Source: three-view drawing plus pictorial views. Frame: mm from the lowest corner of the part. A direction names the side the tool comes from. Coordinates: 2 decimals unless noted, no trailing zeros. Order: outer loops, then holes, each group sorted by start corner. A loop starts at its lowest first (then second) coordinate and runs counter-clockwise, first axis right, second up. Notation, with made-up numbers: (72, 73.25) -> (130, 73.25) arc R17 cw to (130, 83.25) -> close; hole circle Ø2 at (43.5, 13). An arc over 180 degrees is marked (long way). Use one line per item in the form item = value. Start each with the question number.
1) Ray query, line 1 along Y through (x, z) = (6.25, 9.25) (1 decimal); line 2 along Y through (x, z) = (6.25, 18.25) (1 decimal); line 3 along Y through (x, z) = (1.5, 20.25). Return the intervals inside material, ascending.
2) Section query C-C on x = 22.5. Output: boundary loops of the cut face in (y, z).
3) Section query B-B on z = 15.75. Count the separate pieces of the cut face and the enclosed holes in it, then the cut area to 3 significant figures.
4) Pin query (flat end, axial travel): pin 1 (5 mm diameter, centred on x = 9, y = 4, fed in from +Z); pin 2 (4.5 mm diameter, centred on x = 15.5, z = 17.5, fed in from -Y). Return the tip coordinate at first contact, or that it passes through.
5) Section query A-A on x = 18.25. Output: boundary loops of the cut face in (y, z) (1 decimal).
6) Access query for the marked faces 1, 2 and 3. Directions: +Z, -Z, +X, -X, +Y, -Y. A direction counts if a zero-diameter tool reaches every point of the face in a straight line with its end or side. Return the directions, or none.
7) Section query D-D on y = 7.75. Output: boundary loops of the cut face in (x, z).
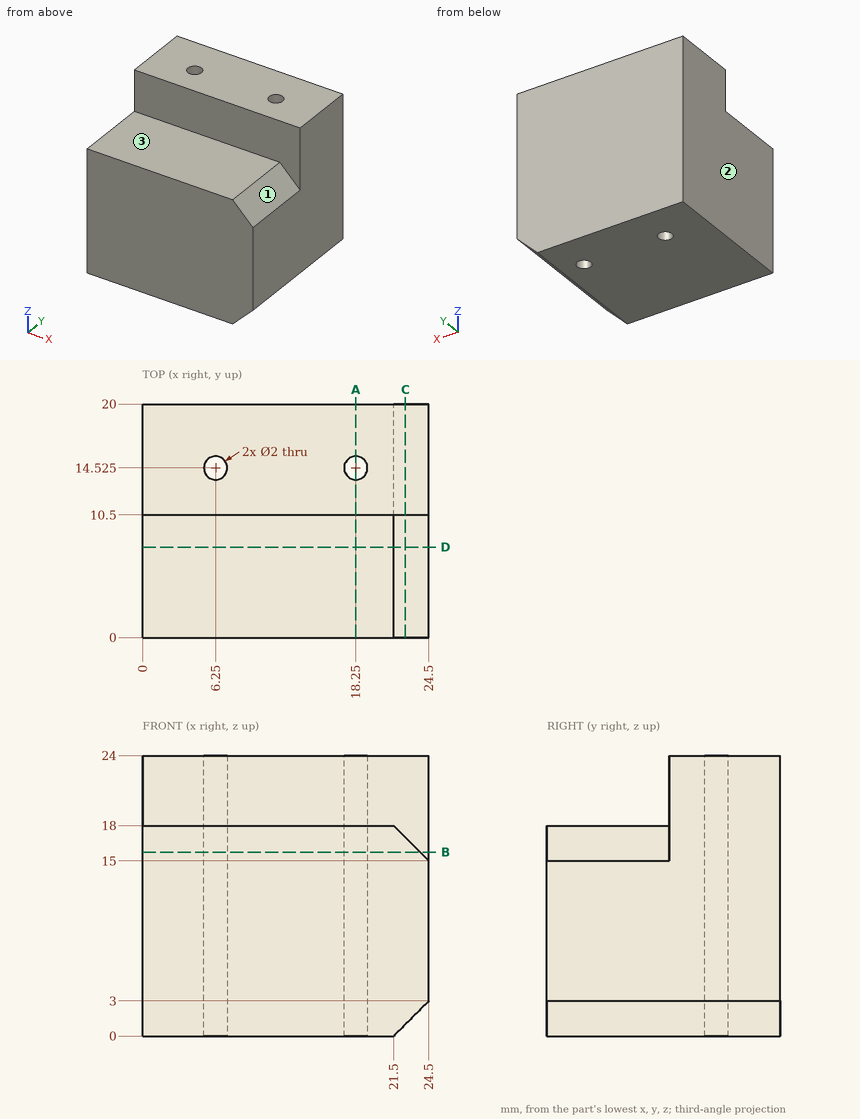
Answers below:
q1.line_1 = 0 to 13.5, 15.5 to 20
q1.line_2 = 10.5 to 13.5, 15.5 to 20
q1.line_3 = 10.5 to 20
q2.outline = (0, 1) -> (20, 1) -> (20, 24) -> (10.5, 24) -> (10.5, 17) -> (0, 17) -> close
q3.separate_pieces = 1
q3.enclosed_holes = 2
q3.area = 476 mm^2
q4.pin_1 = 18
q4.pin_2 = 0
q5.outline = (0, 0) -> (13.5, 0) -> (13.5, 24) -> (10.5, 24) -> (10.5, 18) -> (0, 18) -> close; (15.5, 0) -> (20, 0) -> (20, 24) -> (15.5, 24) -> close
q6.face_1 = +Z, +X, -Y
q6.face_2 = +Z, -Z, -X, +Y, -Y
q6.face_3 = +Z, +X, -X, -Y
q7.outline = (0, 0) -> (21.5, 0) -> (24.5, 3) -> (24.5, 15) -> (21.5, 18) -> (0, 18) -> close
